```python
from build123d import *

# Parameters (mm, degrees)
BOSS_EXTRUDE1_DEPTH = 120.65
SKETCH2_R           = 1.397
CUT_EXTRUDE1_DEPTH  = 129.616537105
SKETCH3_W           = 25.4
SKETCH3_H           = 5.08
CUT_EXTRUDE2_DEPTH  = 129.616537105
SKETCH5_W           = 25.4
SKETCH5_H           = 10.16
BOSS_EXTRUDE3_DEPTH = 3.81
SKETCH6_W           = 8.89
SKETCH6_H           = 63.5
CUT_EXTRUDE3_DEPTH  = 129.616537105
SKETCH7_R           = 4
CUT_EXTRUDE4_DEPTH  = 2
SKETCH8_R           = 4
CUT_EXTRUDE5_DEPTH  = 2


with BuildPart() as part:
    # Sketch1 → Boss-Extrude1 (new body)
    with BuildSketch(Plane.XY):
        Polygon((-40.203883769, 5.937788296), (40.203883769, 5.937788296), (44.399042974, 2.127788296), (-44.399042974, 2.127788296), align=None)
    extrude(amount=BOSS_EXTRUDE1_DEPTH)

    # Sketch2 → Cut-Extrude1 (cut, through all)
    with BuildSketch(Plane.XZ.offset(-2.127788296)):
        with Locations(Location((-31.369, 81.429995649, 0), (0, 0, 270))):
            Circle(SKETCH2_R)
        with Locations(Location((17.653, 23.517995649, 0), (0, 0, 270))):
            Circle(SKETCH2_R)
        with Locations(Location((-31.369, 23.517995649, 0), (0, 0, 270))):
            Circle(SKETCH2_R)
        with Locations(Location((17.653, 81.429995649, 0), (0, 0, 270))):
            Circle(SKETCH2_R)
    extrude(amount=-CUT_EXTRUDE1_DEPTH, mode=Mode.SUBTRACT)

    # Sketch3 → Cut-Extrude2 (cut, through all)
    with BuildSketch(Plane.XZ.offset(-2.127788296)):
        with Locations((0, 118.11)):
            Rectangle(SKETCH3_W, SKETCH3_H)
        with Locations((0, 2.54)):
            Rectangle(SKETCH3_W, SKETCH3_H)
    extrude(amount=-CUT_EXTRUDE2_DEPTH, mode=Mode.SUBTRACT)

    # Sketch5 → Boss-Extrude3 (add)
    with BuildSketch(Plane.XZ.offset(-2.127788296)):
        Rectangle(SKETCH5_W, SKETCH5_H)
    extrude(amount=-BOSS_EXTRUDE3_DEPTH)

    # Sketch6 → Cut-Extrude3 (cut, through all)
    with BuildSketch(Plane.XZ.offset(-2.127788296)):
        with Locations((32.334042974, 64.77)):
            Rectangle(SKETCH6_W, SKETCH6_H)
    extrude(amount=-CUT_EXTRUDE3_DEPTH, mode=Mode.SUBTRACT)

    # Sketch7 → Cut-Extrude4 (cut)
    with BuildSketch(Plane(origin=(21.127225221, 23.263011377, 0), x_dir=(0.7402720771062566, -0.6723074087475077, 0), z_dir=(0.6723074087475077, 0.7402720771062566, 0))):
        with Locations((28.603318705, -90.297)):
            Circle(SKETCH7_R)
        with Locations((28.603318705, -30.353)):
            Circle(SKETCH7_R)
    extrude(amount=-CUT_EXTRUDE4_DEPTH, mode=Mode.SUBTRACT)

    # Sketch8 → Cut-Extrude5 (cut)
    with BuildSketch(Plane(origin=(-21.127225221, 23.263011377, 0), x_dir=(0.7402720771062566, 0.6723074087475077, 0), z_dir=(-0.6723074087475077, 0.7402720771062566, 0))):
        with Locations((-28.603318705, -30.353)):
            Circle(SKETCH8_R)
        with Locations((-28.603318705, -90.297)):
            Circle(SKETCH8_R)
    extrude(amount=-CUT_EXTRUDE5_DEPTH, mode=Mode.SUBTRACT)


solid = part.part
```
CAD build for the part. Positions are in the model's coordinates, mm. A direction names the side the tool comes from. Round coordinates to 2 decimals unless told otherwise and drop trailing zeros. Order: outer loops, then holes, each group sorted by start corner. A loop starts at its lowest first (then second) coordinate and runs counter-clockwise, first axis right, second up. Notation, with made-up numbers: (-38.5, 42) -> (1.5, 42) arc R16 ccw to (1.5, 49) -> close; hole circle Ø6 at (28, -9.5). An arc over 180 degrees is marked (long way). One line per question, with ' | ' between items.
Q1. Slice it at D-D (y = 3.2). Give the number of separate pieces and of enclosed holes in the cut face, then the cut area to 3 significant figures.
Completed:
separate pieces: 1 | enclosed holes: 5 | area: 9,750 mm^2
Q2. Slice it at A-A (z = 44.5). Write the cut outline in (x, y), then the cut area to 3 significant figures.
Completed:
outline: (-44.4, 2.13) -> (27.89, 2.13) -> (27.89, 5.94) -> (-40.2, 5.94) -> close; (36.78, 2.13) -> (44.4, 2.13) -> (40.2, 5.94) -> (36.78, 5.94) -> close | area: 288 mm^2
Q3. Slice it at C-C (z = 19). Write the cut outline in (x, y).
Completed:
outline: (-44.4, 2.13) -> (44.4, 2.13) -> (40.2, 5.94) -> (-40.2, 5.94) -> close
Q4. Drop flat-ended pins along their axis: pin 1 (1.1 mm diameter, centred on y = 3.5, z = 69, fed in from +X); pin 2 (2 mm diameter, centred on y = 4, z = 35, fed in from +X); pin 3 (1.9 mm diameter, centred on x = 4.5, y = 4, fed in from +Z); pin 4 (4.5 mm diameter, centred on x = 17.65, z = 81.43, fed in from -Y). Give the stop position or say it passes through.
Completed:
pin 1: stops at x = 43.49 | pin 2: stops at x = 43.44 | pin 3: stops at z = 115.57 | pin 4: stops at y = 2.13
Q5. Probe probe 1 along Z at (x, y) = (17.5, 5); probe 2 along Z at (x, y) = (28, 2.85); probe 3 along X at (y, z) = (4.85, 60). List the from-to ranges inside material, lowest first.
Completed:
probe 1: z = 0 to 22.13, 24.91 to 80.04, 82.82 to 120.65 | probe 2: z = 0 to 33.02, 96.52 to 120.65 | probe 3: x = -41.4 to 27.89, 36.78 to 41.4
Q6. Two-plate mould, pull along X, no slides. Class faces 4 (the cylindrical face through (-38.38, 5.66, 30.49)), 5 (the flat face through (42.27, 4.06, 59.94)), 6 (the flat face through (-12.7, 4, -3)), 7 (the flat face through (-28, 4, 0)): released by +X, released by -X, zero draft, split by the parting line, or undercut.
Completed:
face 4: undercut | face 5: released by +X | face 6: released by -X | face 7: zero draft
Q7. Slice it at B-B (x = 32.5). Write the cut outline in (y, z), then the cut area to 3 significant figures.
Completed:
outline: (2.13, 0) -> (5.94, 0) -> (5.94, 33.02) -> (2.13, 33.02) -> close; (2.13, 96.52) -> (5.94, 96.52) -> (5.94, 120.65) -> (2.13, 120.65) -> close | area: 218 mm^2
Q8. Which spindle directions (+Z, -Z, +X, -X, +Y, -Y) get a long thin tool onto all of the face, cutting with end or side? Do faces 1 (the flat face through (32, 4, 33.02)), 2 (the flat face through (29, 4, 0)), 3 (the flat face through (0, 4, 115.57)). Say none if no direction does.
Completed:
face 1: +Y, -Y | face 2: -Z, +X, +Y, -Y | face 3: +Z, +Y, -Y
